```python
from build123d import *

# Parameters (mm, degrees)
F2_R     = 24.765
F2_R_2   = 21.082
F4_SIZE2 = 1.27
F4_SIZE  = 4.7397045256
F5_SIZE2 = 1.27
F5_SIZE  = 4.7397045256


with BuildPart() as f3:
    # F3: sweep along a path in F0
    with BuildLine(Plane.XZ) as f3_path:
        Line((0, -42.0079988722), (0, -10.3106039946))
        ThreePointArc((0, -10.3106039946), (1.8947906767, -0.7848479962), (7.2906980027, 7.2906980027))
        Line((7.2906980027, 7.2906980027), (29.7041408666, 29.7041408666))
    # F2 (on plane+point) → F3 (sweep)
    with BuildSketch(Plane.XY.offset(-42.0079988722)):
        Circle(F2_R)
        Circle(F2_R_2, mode=Mode.SUBTRACT)
    sweep(path=f3_path.line)

    # F4
    f4_edges = [f3.edges().sort_by_distance(p)[0] for p in [
        (12.192641, 0, 47.21564),
    ]]
    f4_side = f3.faces().sort_by_distance((0.98592, 0, 36.008919))[0]
    chamfer(f4_edges, length=F4_SIZE, length2=F4_SIZE2, reference=f4_side)

    # F5
    f5_edges = [f3.edges().sort_by_distance(p)[0] for p in [
        (-24.765, 0, -42.007999),
    ]]
    f5_side = f3.faces().sort_by_distance((-24.765, 0, -26.159301))[0]
    chamfer(f5_edges, length=F5_SIZE, length2=F5_SIZE2, reference=f5_side)


solid = f3.part
```
Source: CAD feature listing. Evaluate the final solid. Frame: model axes, mm. A direction names the side the tool comes from. Round coordinates to 2 decimals unless told otherwise and drop trailing zeros. Order: outer loops, then holes, each group sorted by start corner. A loop starts at its lowest first (then second) coordinate and runs counter-clockwise, first axis right, second up. Notation, with made-up numbers: (-24.5, 63.5) -> (9.5, 63.5) arc R18 cw to (9.5, 88.5) -> close; hole circle Ø2 at (-33, 44.25). An arc over 180 degrees is marked (long way). One line per item, written item: value. Start each with the question number.
Q1. Section query A-A (y = 0). Return the cut outline in (x, z) (3 decimals), plus the area to 3 significant figures.
Q2. Pin query (flat end, axial travel): pin 1 (4 mm diameter, centred on y = -6, z = -2, fed in from +X); pin 2 (12 mm diameter, centred on x = -4.5, z = 21, fed in from -Y); pin 3 (1 mm diameter, centred on y = 13.5, z = -18, fed in from +X). Return the tip coordinate at first contact, or that it passes through.
Q3. Draft query along Y for faces 3 (the conical face through (-5.107, -22.996, -41.778)), 4 (the flat face through (42.09, 12.07, 17.32)), 5 (the cylindrical face through (20.11, 6.33, -25.94)). Return one class per face: pulls with the +Y half, pulls with the -Y half, needs draft (parallel to the pull), parting line crosses it, or undercut.
Q4. Material intervals for probe 1 along Y at (x, z) = (0, -21) (3 decimals); probe 2 along X at (y, z) = (6.5, -10); probe 3 along Y at (x, z) = (6.5, 8.5), sorted ascending.
Q5. Access query for faces 1 (the flat face through (-4, -21, -42.008)), 2 (the cylindrical face through (23.62, 7.44, -23.6)). Directions: +Z, -Z, +X, -X, +Y, -Y. A direction counts if a zero-diameter tool reaches every point of the face in a straight line with its end or side. Return the directions, or none.
Findings below:
1. outline: (-24.765, -37.268) -> (-23.495, -42.008) -> (-21.082, -42.008) -> (-21.082, -10.311) arc R45.974 cw to (-7.617, 22.198) -> (14.797, 44.611) -> (13.091, 46.318) -> (8.841, 43.864) -> (-10.221, 24.802) arc R49.657 ccw to (-24.765, -10.311) -> close; (21.082, -42.008) -> (23.495, -42.008) -> (24.765, -37.268) -> (24.765, -10.311) arc R0.127 cw to (24.802, -10.221) -> (43.864, 8.841) -> (46.318, 13.091) -> (44.611, 14.797) -> (22.198, -7.617) arc R3.81 ccw to (21.082, -10.311) -> close
1. area: 599 mm²
2. pin 1: x = 34.09
2. pin 2: y = -21.65
2. pin 3: x = 21.08
3. face 3: parting line crosses it
3. face 4: needs draft
3. face 5: undercut
4. probe 1: -24.765 to -21.082, 21.082 to 24.765
4. probe 2: -23.9 to -20.05, 20.06 to 23.95
4. probe 3: -24.72 to -21.03, 21.03 to 24.72
5. face 1: -Z, +X, -X, +Y, -Y
5. face 2: -Z
